from build123d import *

# Parameters (mm, degrees)
EXTRUDE_1_DEPTH = 10
SKETCH_2_R      = 1.5
EXTRUDE_2_DEPTH = 8
SKETCH_3_W      = 16.5
SKETCH_3_H      = 10
EXTRUDE_3_DEPTH = 8
SKETCH_4_R      = 11
SKETCH_4_R_2    = 5
EXTRUDE_4_DEPTH = 2


with BuildPart() as part:
    # Эскиз1 → Бобышка-Вытянуть1 (new, symmetric)
    with BuildSketch(Plane(origin=(0, 0, 0), x_dir=(1, 0, 0), z_dir=(0, 1, 0))):
        Polygon((-13.25, 21.25), (-21.25, 13.25), (-21.25, -13.25), (-13.25, -21.25), (13.25, -21.25), (21.25, -13.25), (21.25, 13.25), (13.25, 21.25), align=None)
    extrude(amount=EXTRUDE_1_DEPTH, both=True)

    # Эскиз2 → Бобышка-Вытянуть2 (add)
    with BuildSketch(Plane(origin=(0, 10, 0), x_dir=(1, 0, 0), z_dir=(0, 1, 0))):
        Polygon((-17.25, 21.25), (-21.25, 17.25), (-21.25, -17.25), (-17.25, -21.25), (17.25, -21.25), (21.25, -17.25), (21.25, 17.25), (17.25, 21.25), align=None)
        with Locations(Location((-15.5, 15.5, 0), (0, 0, 270))):
            Circle(SKETCH_2_R, mode=Mode.SUBTRACT)
        with Locations(Location((15.5, 15.5, 0), (0, 0, 90))):
            Circle(SKETCH_2_R, mode=Mode.SUBTRACT)
        with Locations(Location((15.5, -15.5, 0), (0, 0, 270))):
            Circle(SKETCH_2_R, mode=Mode.SUBTRACT)
        with Locations(Location((-15.5, -15.5, 0), (0, 0, 90))):
            Circle(SKETCH_2_R, mode=Mode.SUBTRACT)
    extrude_2 = extrude(amount=EXTRUDE_2_DEPTH)

    # Зеркальное отражение1: Бобышка-Вытянуть2 across plane
    add(extrude_2.mirror(Plane.ZX))

    # Эскиз3 → Бобышка-Вытянуть3 (add)
    with BuildSketch(Plane(origin=(0, 0, -21.25), x_dir=(-1, 0, 0), z_dir=(0, 0, -1))):
        with Locations((0, -13)):
            Rectangle(SKETCH_3_W, SKETCH_3_H)
    extrude(amount=EXTRUDE_3_DEPTH)

    # Эскиз4 → Бобышка-Вытянуть4 (add)
    with BuildSketch(Plane(origin=(0, 18, 0), x_dir=(1, 0, 0), z_dir=(0, 1, 0))):
        with Locations(Location((0, 0, 0), (0, 0, 270))):
            Circle(SKETCH_4_R)
        with Locations(Location((0, 0, 0), (0, 0, 270))):
            Circle(SKETCH_4_R_2, mode=Mode.SUBTRACT)
    extrude(amount=EXTRUDE_4_DEPTH)


solid = part.part
For this review, take the finished solid that the model builds, in its own axes (mm). A direction names the side the tool comes from. Round coordinates to 2 decimals unless told otherwise and drop trailing zeros. Loops run counter-clockwise (first coordinate to the right, second up) from the corner with the lowest first, then second, coordinate; pieces in that order, holes last. Notation, with made-up numbers: (6.5, 70.25) - (19.5, 70.25) arc R21 cw to (19.5, 97.25) - close; hole circle Ø3 at (77.25, -25.5). An arc over 180 degrees is marked (long way). One line per question, with ' | ' between items.
Q1. Take a section at C-C (x = -15.5). Give the boundary of the cut face in (y, z), and give its area (3 significant figures).
Taken from the geometry:
outline: (-18, -21.25) - (-10, -21.25) - (-10, -19) - (10, -19) - (10, -21.25) - (18, -21.25) - (18, -17) - (10, -17) - (10, -14) - (18, -14) - (18, 14) - (10, 14) - (10, 17) - (18, 17) - (18, 21.25) - (10, 21.25) - (10, 19) - (-10, 19) - (-10, 21.25) - (-18, 21.25) - (-18, 17) - (-10, 17) - (-10, 14) - (-18, 14) - (-18, -14) - (-10, -14) - (-10, -17) - (-18, -17) - close | area: 1,340 mm²
Q2. For line 1 along X through (y, z) = (-15, -15.5); line 2 along X through (y, z) = (-13, -15); line 3 along X through (y, z) = (19.3, 0), list the stretches that pass through material, from the lowest coordinate up. Write a range as [from, to].
Taken from the geometry:
line 1: x = [-21.25, -17], [-14, 14], [17, 21.25] | line 2: x = [-21.25, -16.91], [-14.09, 14.09], [16.91, 21.25] | line 3: x = [-11, -5], [5, 11]
Q3. Take a section at D-D (y = -15). Give the boundary of the cut face in (x, z), and give its area (3 significant figures).
Taken from the geometry:
outline: (-21.25, -17.25) - (-17.25, -21.25) - (-8.25, -21.25) - (-8.25, -29.25) - (8.25, -29.25) - (8.25, -21.25) - (17.25, -21.25) - (21.25, -17.25) - (21.25, 17.25) - (17.25, 21.25) - (-17.25, 21.25) - (-21.25, 17.25) - close; hole circle Ø3 at (-15.5, -15.5); hole circle Ø3 at (-15.5, 15.5); hole circle Ø3 at (15.5, -15.5); hole circle Ø3 at (15.5, 15.5) | area: 1,880 mm²
Q4. Take a section at A-A (y = 16). Give the boundary of the cut face in (x, z), and give its area (3 significant figures).
Taken from the geometry:
outline: (-21.25, -17.25) - (-17.25, -21.25) - (17.25, -21.25) - (21.25, -17.25) - (21.25, 17.25) - (17.25, 21.25) - (-17.25, 21.25) - (-21.25, 17.25) - close; hole circle Ø3 at (-15.5, -15.5); hole circle Ø3 at (-15.5, 15.5); hole circle Ø3 at (15.5, -15.5); hole circle Ø3 at (15.5, 15.5) | area: 1,750 mm²
Q5. Take a section at B-B (z = -15.5). Give the boundary of the cut face in (x, y), and give its area (3 significant figures).
Taken from the geometry:
outline: (-21.25, -18) - (-17, -18) - (-17, -10) - (-14, -10) - (-14, -18) - (14, -18) - (14, -10) - (17, -10) - (17, -18) - (21.25, -18) - (21.25, -10) - (19, -10) - (19, 10) - (21.25, 10) - (21.25, 18) - (17, 18) - (17, 10) - (14, 10) - (14, 18) - (-14, 18) - (-14, 10) - (-17, 10) - (-17, 18) - (-21.25, 18) - (-21.25, 10) - (-19, 10) - (-19, -10) - (-21.25, -10) - close | area: 1,340 mm²
Q6. The part is to be moulded in two halves that separate along Z. For faces 5 (the cylindrical face through (-15.43, -13.94, -17)), 6 (the flat face through (17.3, 0.1, -17.2)), 7 (the cylindrical face through (-10.74, 18.99, -2.38)), 8 (the cylindrical face through (-4.88, 18.99, -1.08)), say which applies: released by +Z, released by -Z, zero draft, split by the parting line, or undercut.
Taken from the geometry:
face 5: undercut | face 6: released by -Z | face 7: split by the parting line | face 8: undercut
Q7. For pin 1 (6 mm diameter, centred on x = -13.5, y = 10, fed in from -Z); pin 2 (6.5 mm diameter, centred on x = 16, z = 18.5, fed in from +Y); pin 3 (2.5 mm diameter, centred on x = -15.5, z = -15.5, fed in from +Y), all flat-tipped, find the tip position at first contact; note any pin that passes through.
Taken from the geometry:
pin 1: stops at z = -21.25 | pin 2: stops at y = 18 | pin 3: stops at y = 10
Q8. Tool access review of faces 1 (the flat face through (-18, 10, 18)), 2 (the flat face through (18, -10, -18)), 3 (the flat face through (-16, -10, 15)), 4 (the flat face through (17.2, 0.1, 17.3)): name each direction out of +Z, -Z, +X, -X, +Y, -Y from which nothing blocks a thin tool from reaching the whole face with its end or side.
Taken from the geometry:
face 1: +Z, -X | face 2: -Z, +X | face 3: -Y | face 4: +Z, +X
